```python
from build123d import *

# Parameters (mm, degrees)
F0_R     = 20.25
F0_R_2   = 18.75
F1_DEPTH = 23
F0_R_3   = 0.75
F2_DEPTH = 2
F3_R     = 0.7
F4_SIZE2 = 1.5
F4_SIZE  = 1.5


with BuildPart() as f1:
    # F0 (on Top) → F1 (new body)
    with BuildSketch(Plane.XY):
        Circle(F0_R)
        Circle(F0_R_2, mode=Mode.SUBTRACT)
    extrude(amount=F1_DEPTH)

    # F0 (on Top) → F2 (join)
    with BuildSketch(Plane.XY):
        Circle(F0_R_2)
        Circle(F0_R_3, mode=Mode.SUBTRACT)
    extrude(amount=F2_DEPTH)

    # F3
    f3_edges = [f1.edges().sort_by_distance(p)[0] for p in [
        (-20.25, 0, 23),
        (-18.75, 0, 23),
        (-20.25, 0, 0),
    ]]
    fillet(f3_edges, radius=F3_R)

    # F4
    f4_edges = [f1.edges().sort_by_distance(p)[0] for p in [
        (-0.75, 0, 0),
    ]]
    chamfer(f4_edges, length=F4_SIZE, length2=F4_SIZE2)


solid = f1.part
```
Geometry: final body of the model. Coordinates: model frame, mm. A direction names the side the tool comes from. Round coordinates to 2 decimals unless told otherwise and drop trailing zeros. Loops run counter-clockwise (first coordinate to the right, second up) from the corner with the lowest first, then second, coordinate; pieces in that order, holes last. Notation, with made-up numbers: (25.25, 17) -> (62.25, 17) arc R16 ccw to (62.25, 36) -> close; hole circle Ø4 at (8, 6.5). An arc over 180 degrees is marked (long way). Use one line per item in the form item = value.
Item 1: Access query for faces 1 (the cylindrical face through (-0.75, 0.03, 1.75)), 2 (the cylindrical face through (-2.44, 18.59, 12.01)). Directions: +Z, -Z, +X, -X, +Y, -Y. A direction counts if a zero-diameter tool reaches every point of the face in a straight line with its end or side. Return the directions, or none.
Evaluation:
face_1 = +Z, -Z
face_2 = +Z
Item 2: Material intervals for probe 1 along Y at (x, z) = (0, 11.5); probe 2 along X at (y, z) = (0.5, 7.75); probe 3 along Y at (x, z) = (4.5, 12), sorted ascending.
Evaluation:
probe_1 = -20.25 to -18.75, 18.75 to 20.25
probe_2 = -20.24 to -18.74, 18.74 to 20.24
probe_3 = -19.74 to -18.2, 18.2 to 19.74
Item 3: Draft query along X for faces 3 (the cylindrical face through (11, 17, 11)), 4 (the flat face through (4, 0, 2)), 5 (the flat face through (0, -4, 0)). Return one class per face: released by +X, released by -X, zero draft, split by the parting line, or undercut.
Evaluation:
face_3 = split by the parting line
face_4 = undercut
face_5 = zero draft
Item 4: Cut plane A-A on x = 0. Output: boundary loops of the cut face in (y, z).
Evaluation:
outline = (-20.25, 0.7) arc R0.7 ccw to (-19.55, 0) -> (-2.25, 0) -> (-0.75, 1.5) -> (-0.75, 2) -> (-18.75, 2) -> (-18.75, 22.3) arc R0.7 ccw to (-19.45, 23) -> (-19.55, 23) arc R0.7 ccw to (-20.25, 22.3) -> close; (0.75, 1.5) -> (2.25, 0) -> (19.55, 0) arc R0.7 ccw to (20.25, 0.7) -> (20.25, 22.3) arc R0.7 ccw to (19.55, 23) -> (19.45, 23) arc R0.7 ccw to (18.75, 22.3) -> (18.75, 2) -> (0.75, 2) -> close
Item 5: Contact query for flat-ended pins moving along their axis: pin 1 Ø6 at (x, y) = (-3.5, 4) entering from +Z; pin 2 Ø12 at (x, z) = (-3, 2.5) entering from -Y; pin 3 Ø1 at (y, z) = (7.5, 5.5) entering from -X. Output: stop coordinate, or through.
Evaluation:
pin_1 = 2
pin_2 = -20.25
pin_3 = -19
Item 6: Cut plane C-C on z = 10. Output: boundary loops of the cut face in (x, y).
Evaluation:
outline = circle Ø40.5 at (0, 0); hole circle Ø37.5 at (0, 0)
